Build history of the part. All positions in model axes, mm. Face numbers are marked on the shaded views. Give positions to 0.01 mm unless a question says otherwise; leave off trailing zeros. Loops run counter-clockwise (first coordinate to the right, second up) from the corner with the lowest first, then second, coordinate; pieces in that order, holes last.
1) Band-saw the part on D-D on y = 5. State how many separate pieces and enclosed holes the cut face has, then the cut area to 3 significant figures.
2) Band-saw the part on C-C on z = -58.5. List the corners of the cut face in (x, y), then the cut area to 3 significant figures.
3) Wall check: line 1 (X direction, y = 15.5, z = 0); line 2 (Y direction, x = 95, z = -97.1); line 3 (X direction, y = 6, z = -33.5). Give the ranges that are in metal, low to high.
4) Band-saw the part on B-B on x = 0. List the corners of the cut face in (y, z), then the cut area to 3 significant figures.
5) Two-plate mould, pull along X, no slides. Class the marked faces 1 and 2: +X half, -X half, draft (parallel to the pull), parting line (faces both ways), or undercut.
6) Band-saw the part on A-A on z = 0. List the corners of the cut face in (x, y), then the cut area to 3 significant figures.
7) Flat gauge pin, fed straight in: P1, Ø5, axis at y = 13.5, z = -88, coming from the +X side. Where does the tip first touch, or does it go through?
```python
from build123d import *

# Parameters (mm, degrees)
ESQUISSE1_R             = 15
BASE_DEPTH              = 20
ESQUISSE2_R             = 2.5
ENL_V_MAT_EXTRU_1_DEPTH = 225.499443206


with BuildPart() as part:
    # Esquisse1 → BASE (new body)
    with BuildSketch(Plane(origin=(0, 0, 0), x_dir=(1, 0, 0), z_dir=(0, 1, 0))):
        Polygon((-100, 95), (-90, 95), (-90, 85), (-100, 85), (-100, -85), (-90, -85), (-90, -95), (-100, -95), (-100, -100), (100, -100), (100, -95), (90, -95), (90, -85), (100, -85), (100, 85), (90, 85), (90, 95), (100, 95), (100, 100), (-100, 100), align=None)
        with Locations(Location((0, 0, 0), (0, 0, 270))):
            Circle(ESQUISSE1_R, mode=Mode.SUBTRACT)
    extrude(amount=BASE_DEPTH)

    # Esquisse2 → Enlèv. mat.-Extru.1 (cut, through all)
    with BuildSketch(Plane.XY.offset(100)):
        with Locations((-95, 15)):
            Circle(ESQUISSE2_R)
        with Locations((-95, 5)):
            Circle(ESQUISSE2_R)
        with Locations(Location((95, 5, 0), (0, 0, 180))):
            Circle(ESQUISSE2_R)
        with Locations(Location((95, 15, 0), (0, 0, 180))):
            Circle(ESQUISSE2_R)
    extrude(amount=-ENL_V_MAT_EXTRU_1_DEPTH, mode=Mode.SUBTRACT)


solid = part.part
```
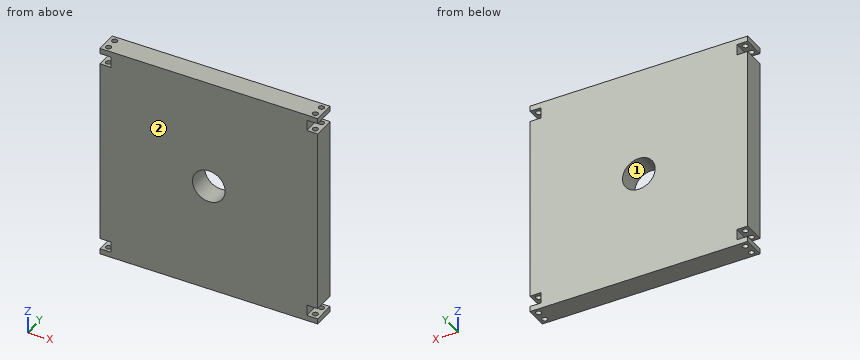
Findings below:
1. separate pieces: 7
1. enclosed holes: 1
1. area: 37,100 mm2
2. outline: (-100, 0) - (100, 0) - (100, 20) - (-100, 20) - close; hole circle Ø5 at (-95, 5); hole circle Ø5 at (-95, 15); hole circle Ø5 at (95, 5); hole circle Ø5 at (95, 15)
2. area: 3,920 mm2
3. line 1: x = -100 to -97.45, -92.55 to -15, 15 to 92.55, 97.45 to 100
3. line 2: y = 0 to 2.5, 7.5 to 12.5, 17.5 to 20
3. line 3: x = -100 to -97.29, -92.71 to 92.71, 97.29 to 100
4. outline: (0, -100) - (20, -100) - (20, -15) - (0, -15) - close; (0, 15) - (20, 15) - (20, 100) - (0, 100) - close
4. area: 3,400 mm2
5. face 1: undercut
5. face 2: draft
6. outline: (-100, 0) - (-15, 0) - (-15, 20) - (-100, 20) - close; (15, 0) - (100, 0) - (100, 20) - (15, 20) - close; hole circle Ø5 at (-95, 5); hole circle Ø5 at (-95, 15); hole circle Ø5 at (95, 5); hole circle Ø5 at (95, 15)
6. area: 3,320 mm2
7. P1: stops at x = 90
